```python
from build123d import *

# Parameters (mm, degrees)
SKETCH2_W                 = 5
SKETCH2_H                 = 1.5
LPATTERN1_COUNT           = 10
LPATTERN1_PITCH           = 2.5
M7X1_0_TAPPED_HOLE1_D     = 6
M7X1_0_TAPPED_HOLE1_DEPTH = 15.1
M7X1_0_TAPPED_HOLE1_TIP   = 1.802581857


with BuildPart() as part:
    # Sketch1 → Revolve1 (revolve)
    with BuildSketch(Plane.XY):
        Polygon((0, 42.7), (0, 0), (11.15, 0), (11.15, 1), (11, 1), (11, 26), (3.5, 26), (3.5, 27.5), (8, 27.5), (8, 28.5), (3.5, 28.5), (3.5, 30), (8, 30), (8, 33), (6, 33), (6, 39), (8, 39), (8, 42.7), align=None)
    revolve(axis=Axis((0, 0, 0), (0, -1, 0)))

    # Sketch2 → Cut-Revolve1 (revolve, cut)
    with BuildSketch(Plane.XY):
        with Locations((8.5, 1.75)):
            Rectangle(SKETCH2_W, SKETCH2_H)
    cut_revolve1 = revolve(axis=Axis((0, 0, 0), (0, 1, 0)), mode=Mode.SUBTRACT)

    # LPattern1: Cut-Revolve1 ×10
    with Locations(*[(0, i * LPATTERN1_PITCH, 0) for i in range(1, LPATTERN1_COUNT)]):
        add(cut_revolve1, mode=Mode.SUBTRACT)

    # Sketch3 → Cut-Revolve2 (revolve, cut)
    with BuildSketch(Plane.XY):
        Polygon((0, 42.7), (0, 0), (2.1, 0), (2.1, 34.3), (4, 36.2), (4, 42.7), align=None)
    revolve(axis=Axis((0, 42.7, 0), (0, -1, 0)), mode=Mode.SUBTRACT)

    # M7x1.0 Tapped Hole1
    with Locations(Plane(origin=(0, 0, 0), x_dir=(-1, 0, 0), z_dir=(0, -1, 0))):
        with Locations((0, 0)):
            Hole(M7X1_0_TAPPED_HOLE1_D / 2, depth=M7X1_0_TAPPED_HOLE1_DEPTH)
            with Locations((0, 0, -(M7X1_0_TAPPED_HOLE1_DEPTH + M7X1_0_TAPPED_HOLE1_TIP / 2))):  # 118° drill point
                Cone(0, M7X1_0_TAPPED_HOLE1_D / 2, M7X1_0_TAPPED_HOLE1_TIP, mode=Mode.SUBTRACT)


solid = part.part
```
The listing builds one solid part. Answer for the finished solid, in the listing's coordinates (mm). A direction names the side the tool comes from. Coordinates: 2 decimals unless noted, no trailing zeros. Write each loop counter-clockwise with the first axis right and the second up, starting at its lowest first coordinate (ties: lowest second). Pieces come first, ordered by that corner, then holes.
Q1. The mould has two halves that part along Y. Classify faces 1 (the cylindrical face through (-6, 24, 0)), 2 (the cylindrical face through (-2.38, 25.51, -10.74)), 3 (the flat face through (-2.3, 0, -2.3)): released by +Y, released by -Y, zero draft, split by the parting line, or undercut.
Returned:
face 1: undercut
face 2: zero draft
face 3: released by -Y
Q2. Find the intervals of material crossed by line 1 along Y through (x, z) = (-3, -4.75); line 2 along Z through (x, y) = (0, 23.75); line 3 along X through (y, z) = (12, 1.5), in increasing order.
Returned:
line 1: y = 0 to 26, 27.5 to 28.5, 30 to 42.7
line 2: z = -6 to -2.1, 2.1 to 6
line 3: x = -5.81 to -2.6, 2.6 to 5.81
Q3. Section D-D, the plane y = 13 is taken. Write down the section's boundary in (x, z).
Returned:
outline: circle Ø22 at (0, 0); hole circle Ø6 at (0, 0)
Q4. Which of the six approach directions +Z, -Z, +X, -X, +Y, -Y give full straight-line access (tool end or side, diameter ignored) to faces 4 (the cylindrical face through (-2.38, 13.01, -10.74)), 5 (the flat face through (-5, 5, 5))?
Returned:
face 4: +Y
face 5: none
Q5. Given P1, Ø12, axis at x = 0.5, y = 26.5, coming from the -Z side; P2, Ø1, axis at y = 25.5, z = 8.5, coming from the -X side; P3, Ø2, axis at y = 8.5, z = -6, coming from the -X side, each flat-ended and moving along its own axis, determine where each tip first touches the part or whether it passes through.
Returned:
P1: stops at z = -11
P2: stops at x = -7.55
P3: stops at x = -9.8
Q6. Section A-A, the plane y = 7 is taken. Write down the section's boundary in (x, z).
Returned:
outline: circle Ø12 at (0, 0); hole circle Ø6 at (0, 0)
Q7. Section B-B, the plane x = -4.75 is taken. Give the number of separate pieces and of enclosed holes in the cut face, then the cut area to 3 significant figures.
Returned:
separate pieces: 3
enclosed holes: 0
area: 472 mm2
